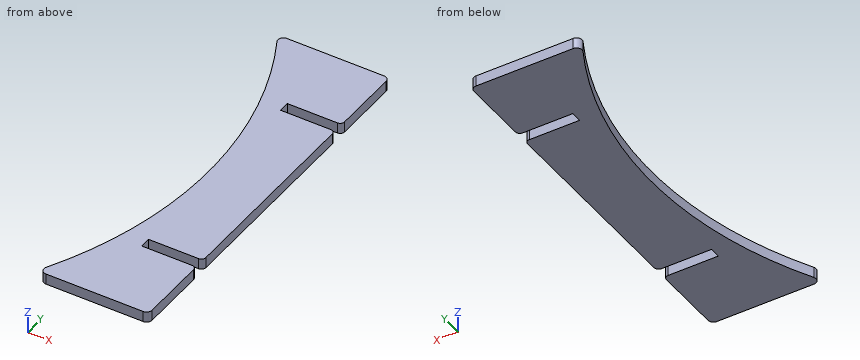
```python
from build123d import *

# Parameters (mm, degrees)
RESSALTO_EXTRUS_O1_DEPTH = 5


with BuildPart() as part:
    # Model → Ressalto-extrusão1 (new body)
    with BuildSketch(Plane.XY):
        with BuildLine():
            Line((8.958908168, 92.500001378), (-14.205034542, 92.500001378))
            Line((-14.205034542, 92.500001378), (-14.205034542, 87.500001303))
            Line((-14.205034542, 87.500001303), (8.958908168, 87.500001303))
            ThreePointArc((8.958908168, 87.500001303), (10.37312173, 86.914214866), (10.958908168, 85.500001303))
            Line((10.958908168, 85.500001303), (10.958908168, -7.500000142))
            ThreePointArc((10.958908168, -7.500000142), (10.37312173, -8.914213705), (8.958908168, -9.500000142))
            Line((8.958908168, -9.500000142), (-14.237425511, -9.500000142))
            Line((-14.237425511, -9.500000142), (-14.237425511, -14.500000217))
            Line((-14.237425511, -14.500000217), (8.958908168, -14.500000217))
            ThreePointArc((8.958908168, -14.500000217), (10.37312173, -15.085786654), (10.958908168, -16.500000217))
            Line((10.958908168, -16.500000217), (10.958908168, -47.000089001))
            ThreePointArc((10.958908168, -47.000089001), (10.226675121, -48.767855954), (8.458908168, -49.500089001))
            Line((8.458908168, -49.500089001), (-36.392181846, -49.500089001))
            ThreePointArc((-36.392181846, -49.500089001), (-38.532153082, -48.292576181), (-38.604890155, -45.836507488))
            ThreePointArc((-38.604890155, -45.836507488), (-17.243723681, 39.000273479), (-38.605225502, 123.836970009))
            ThreePointArc((-38.605225502, 123.836970009), (-38.53196676, 126.292709214), (-36.392181846, 127.499913592))
            Line((-36.392181846, 127.499913592), (8.458908168, 127.499913592))
            ThreePointArc((8.458908168, 127.499913592), (10.226675121, 126.767680545), (10.958908168, 124.999913592))
            Line((10.958908168, 124.999913592), (10.958908168, 94.500001378))
            ThreePointArc((10.958908168, 94.500001378), (10.37312173, 93.085787815), (8.958908168, 92.500001378))
        make_face()
    extrude(amount=RESSALTO_EXTRUS_O1_DEPTH)


solid = part.part
```
Geometry check sheet. Reference: the model listing, model coordinates, mm. Coordinates: 2 decimals unless noted, no trailing zeros. Write each loop counter-clockwise with the first axis right and the second up, starting at its lowest first coordinate (ties: lowest second). Pieces come first, ordered by that corner, then holes. Notation, with made-up numbers: M -29.5,-25.75 L 29.5,-25.75 A22 cw 29.5,-10.75 Z; hole C -20,85 d11. An arc over 180 degrees is marked long. Use one line per item in the form item = value. Start each with the question number.
1) Section check B-B on x = -23. Enter the section's corners in (y, z).
2) Thickness scan on probe 1 along Y at (x, z) = (2.5, 1.6); probe 2 along Y at (x, z) = (-35.5, 4.4); probe 3 along Y at (x, z) = (-31.5, 0.35). Record the ranges inside material, lowest first. Write a range as from..to.
3) Section check A-A on x = 3.5. Enter the section's corners in (y, z).
4) Section check C-C on z = 1. Enter the section's corners in (x, y).
5) Go/stop test with flat-tipped pins: pin 1 Ø1.5 at (y, z) = (-12, 3.5) entering from +X; pin 2 Ø2 at (y, z) = (78.5, 1.5) entering from -X. Record where each tip stops, or that it passes through.
6) Section check D-D on y = 40. Enter the section's corners in (x, z), and give its area (3 significant figures).
Responses:
q1.outline = M -49.5,0 L -6.05,0 L -6.05,5 L -49.5,5 Z; M 84.05,0 L 127.5,0 L 127.5,5 L 84.05,5 Z
q2.probe_1 = -49.5..-14.5, -9.5..87.5, 92.5..127.5
q2.probe_2 = -49.5..-39.79, 117.79..127.5
q2.probe_3 = -49.5..-31.03, 109.03..127.5
q3.outline = M -49.5,0 L -14.5,0 L -14.5,5 L -49.5,5 Z; M -9.5,0 L 87.5,0 L 87.5,5 L -9.5,5 Z; M 92.5,0 L 127.5,0 L 127.5,5 L 92.5,5 Z
q4.outline = M -38.61,123.84 A179.15 cw -38.6,-45.84 A2.5 ccw -36.39,-49.5 L 8.46,-49.5 A2.5 ccw 10.96,-47 L 10.96,-16.5 A2 ccw 8.96,-14.5 L -14.24,-14.5 L -14.24,-9.5 L 8.96,-9.5 A2 ccw 10.96,-7.5 L 10.96,85.5 A2 ccw 8.96,87.5 L -14.21,87.5 L -14.21,92.5 L 8.96,92.5 A2 ccw 10.96,94.5 L 10.96,125 A2.5 ccw 8.46,127.5 L -36.39,127.5 A2.5 ccw Z
q5.pin_1 = -14.24
q5.pin_2 = -21.88
q6.outline = M -17.25,0 L 10.96,0 L 10.96,5 L -17.25,5 Z
q6.area = 141 mm2
